Could you check a few things on this model? Use its own coordinates, in mm. A direction names the side the tool comes from. Round coordinates to 2 decimals unless told otherwise and drop trailing zeros. Write each loop counter-clockwise with the first axis right and the second up, starting at its lowest first coordinate (ties: lowest second). Pieces come first, ordered by that corner, then holes. Notation, with made-up numbers: M 40.5,2 L 86.5,2 A32 ccw 86.5,28 Z; hole C 43,13 d3. An arc over 180 degrees is marked long. One line per item, written item: value. Start each with the question number.
(1) I want a section at C-C on z = 20. Please give me the cut outline in (x, y), and give its area (3 significant figures).
(2) If I drill on L1, parallel to X at y = 77, z = -20; L2, parallel to X at y = 42, z = -12, over which ranges is the centre line in solid material (lowest first)?
(3) Thinking about a two-plate mould opening in Z: for faces 1 (the face through (-22.43, 50.7, 22.4)), 2 (the face through (0, 49, -21)), 3 (the face through (23, 49, -11)), which applies, released by +Z, released by -Z, zero draft, split by the parting line, or undercut?
(4) I'm going to push flat-ended pins straight in: pin 1 Ø3 at (x, z) = (20, -20) entering from +Y; pin 2 Ø2.5 at (x, y) = (8, 50) entering from -Z; pin 3 Ø1.8 at (x, z) = (-20, -20) entering from +Y. Where does each tip first touch, or does it pass through?
(5) I want a section at D-D on x = 17.5. Please give me the cut outline in (y, z).
(6) Which directions (+Z, -Z, +X, -X, +Y, -Y) give clear straight access to the entire face, cutting with the end or side of a thin tool? Please do faces 4 (the face through (0, 49, -23)), 5 (the face through (-21, 49, 0)), 6 (the face through (-7.675, 48.536, -22.014)).
(7) I want a section at B-B on x = -8. Please give me the cut outline in (y, z).
(8) I want a section at A-A on y = 50. Count the separate pieces of the cut face and the enclosed holes in it, and give its area (3 significant figures).
```python
from build123d import *

# Parameters (mm, degrees)
SKETCH1_R           = 1
BOSS_EXTRUDE1_DEPTH = 100
FILLET1_R           = 2
CUT_EXTRUDE2_REACH  = 48
SKETCH3_R           = 1.5
FILLET2_R           = 2


with BuildPart() as part:
    # Sketch1 → Boss-Extrude1 (new body)
    with BuildSketch(Plane(origin=(0, 0, 0), x_dir=(1, 0, 0), z_dir=(0, 1, 0))):
        Polygon((-23, 0.601609353), (-22.074492009, 0), (-23, -0.601609353), (-23, -23), (23, -23), (23, -0.712327005), (22.071835016, 0), (23, 0.712327005), (23, 23), (-23, 23), align=None)
        with Locations((-20, 20)):
            Circle(SKETCH1_R, mode=Mode.SUBTRACT)
        with Locations((20, 20)):
            Circle(SKETCH1_R, mode=Mode.SUBTRACT)
        with Locations((20, -20)):
            Circle(SKETCH1_R, mode=Mode.SUBTRACT)
        with Locations((-20, -20)):
            Circle(SKETCH1_R, mode=Mode.SUBTRACT)
        with BuildLine():
            Line((-18.881966011, 21), (18.881966011, 21))
            ThreePointArc((18.881966011, 21), (18.939339828, 18.939339828), (21, 18.881966011))
            Line((21, 18.881966011), (21, -18.881966011))
            ThreePointArc((21, -18.881966011), (18.939339828, -18.939339828), (18.881966011, -21))
            Line((18.881966011, -21), (-18.881966011, -21))
            ThreePointArc((-18.881966011, -21), (-18.939339828, -18.939339828), (-21, -18.881966011))
            Line((-21, -18.881966011), (-21, 18.881966011))
            ThreePointArc((-21, 18.881966011), (-18.939339828, 18.939339828), (-18.881966011, 21))
        make_face(mode=Mode.SUBTRACT)
    extrude(amount=BOSS_EXTRUDE1_DEPTH)

    # Fillet1
    fillet1_edges = [part.edges().sort_by_distance(p)[0] for p in [
        (-23, 50, -23),
        (23, 50, -23),
    ]]
    fillet(fillet1_edges, radius=FILLET1_R)

    # Sketch3 → Cut-Extrude2 (cut, up to next)
    with BuildSketch(Plane(origin=(0, 0, -23), x_dir=(-1, 0, 0), z_dir=(0, 0, -1)), mode=Mode.PRIVATE) as cut_extrude2_sk1:
        with Locations((8, 50)):
            Circle(SKETCH3_R)
    cut_extrude2_tool1 = extrude(cut_extrude2_sk1.sketch, amount=-CUT_EXTRUDE2_REACH, mode=Mode.PRIVATE) & part.part
    add(cut_extrude2_tool1.solids().sort_by_distance((-8, 50, -23))[0], mode=Mode.SUBTRACT)
    # Sketch3 → Cut-Extrude2 (cut, up to next)
    with BuildSketch(Plane(origin=(0, 0, -23), x_dir=(-1, 0, 0), z_dir=(0, 0, -1)), mode=Mode.PRIVATE) as cut_extrude2_sk2:
        with Locations((-8, 50)):
            Circle(SKETCH3_R)
    cut_extrude2_tool2 = extrude(cut_extrude2_sk2.sketch, amount=-CUT_EXTRUDE2_REACH, mode=Mode.PRIVATE) & part.part
    add(cut_extrude2_tool2.solids().sort_by_distance((8, 50, -23))[0], mode=Mode.SUBTRACT)

    # Fillet2
    fillet2_edges = [part.edges().sort_by_distance(p)[0] for p in [
        (23, 50, 23),
        (-23, 50, 23),
    ]]
    fillet(fillet2_edges, radius=FILLET2_R)


solid = part.part
```
Found:
1. outline: M -23,0 L -21,0 L -21,100 L -23,100 Z; M -19,0 L -18.5,0 L -18.5,100 L -19,100 Z; M 18.5,0 L 19,0 L 19,100 L 18.5,100 Z; M 21,0 L 23,0 L 23,100 L 21,100 Z
1. area: 500 mm²
2. L1: x = -23 to -21, -19 to -18.5, 18.5 to 19, 21 to 23
2. L2: x = -23 to -21, 21 to 23
3. face 1: released by +Z
3. face 2: undercut
3. face 3: zero draft
4. pin 1: stops at y = 100
4. pin 2: stops at z = 21
4. pin 3: passes through
5. outline: M 0,-23 L 100,-23 L 100,-21 L 0,-21 Z; M 0,21 L 100,21 L 100,23 L 0,23 Z
6. face 4: -Z, +X, -X, +Y, -Y
6. face 5: +Y, -Y
6. face 6: -Z
7. outline: M 0,-23 L 48.5,-23 L 48.5,-21 L 0,-21 Z; M 0,21 L 100,21 L 100,23 L 0,23 Z; M 51.5,-23 L 100,-23 L 100,-21 L 51.5,-21 Z
8. separate pieces: 2
8. enclosed holes: 4
8. area: 345 mm²
